Model file for the job. Use its own axes, mm. Face numbers are marked on the shaded views. Round coordinates to 2 decimals unless told otherwise and drop trailing zeros. Loops run counter-clockwise (first coordinate to the right, second up) from the corner with the lowest first, then second, coordinate; pieces in that order, holes last. Notation, with made-up numbers: (40.5, 69.5) - (89.5, 69.5) arc R29 cw to (89.5, 93.5) - close; hole circle Ø9 at (78.25, 79). An arc over 180 degrees is marked (long way). Answer as a JSON object with one key per item and string values.
Solid Edge part; units mm, degrees
sketch "Sketch1" plane through (0, 0, 0) normal (0, 0, 1) x (1, 0, 0)
  line L0 (15, -30) -> (-15, -30)
  line L1 (-15, -30) -> (-15, 30)
  line L2 (-15, 30) -> (15, 30)
  line L3 (15, 30) -> (15, -30)
extrude "Protrusion1" add sketch "Sketch1" against normal blind 5
sketch "Sketch2" plane through (0, -30, -2.5) normal (0, -1, 0) x (1, 0, 0)
  line L0 (15, -2.5) -> (15, -4.45)
  line L1 (15, -4.45) -> (-15, -4.45)
  line L2 (-15, -4.45) -> (-15, -2.5)
  line L3 (-15, -2.5) -> (15, -2.5)
extrude "ExtrudedProtrusion_2" add sketch "Sketch2" against normal blind 15
fillet "Round_1" radius 2 1 edges at (0, -15, -6.95)
sketch "Sketch3" plane through (0, -30, -3.475) normal (0, -1, 0) x (1, 0, 0)
  circle A0 centre (-5.74, -3.475) radius 0.5
  circle A1 centre (-2.87, -3.475) radius 0.5
  circle A2 centre (0, -3.475) radius 0.5
  circle A3 centre (2.87, -3.475) radius 0.5
  circle A4 centre (5.74, -3.475) radius 0.5
extrude "Cutout1" cut sketch "Sketch3" against normal up to next
sketch "Sketch4" plane through (0, 0, 0) normal (0, 0, 1) x (1, 0, 0)
  circle A0 centre (11.5, -25) radius 2.125
  circle A1 centre (-11.5, -25) radius 2.125
  circle A2 centre (-11.5, 25) radius 2.125
  circle A3 centre (11.5, 25) radius 2.125
extrude "Cutout2" cut sketch "Sketch4" against normal up to next
sketch "Sketch5" plane through (0, 7.5, -5) normal (0, 0, -1) x (-1, 0, 0)
  line L0 (3.2448, 10.1167) -> (3.2448, -2.3765)
  line L1 (3.2448, -2.3765) -> (8.2455, -2.3765)
  line L2 (8.2455, -2.3765) -> (8.2455, 10.1167)
  line L3 (8.2455, 10.1167) -> (3.2448, 10.1167)
extrude "Cutout3" cut sketch "Sketch5" against normal up to next
sketch "Sketch6" plane through (15, 0, -3.475) normal (1, 0, 0) x (0, 1, 0)
  line L0 (-15, -1.525) -> (-14.875, 3.475)
  line L1 (-14.875, 3.475) -> (30, 3.475)
  line L2 (30, 3.475) -> (30, -1.525)
  line L3 (30, -1.525) -> (-15, -1.525)
extrude "Cutout4" cut sketch "Sketch6" against normal up to next
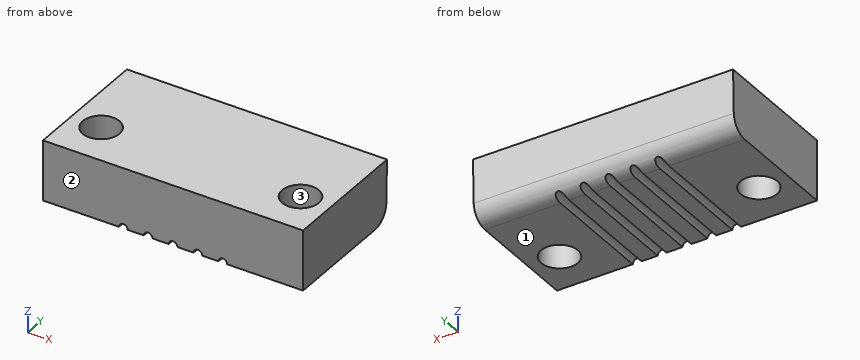
1) Two-plate mould, pull along Y, no slides. Class the marked faces 1, 2 and 3: pulls with the +Y half, pulls with the -Y half, needs draft (parallel to the pull), parting line crosses it, or undercut.
Values follow:
{"face 1": "needs draft", "face 2": "pulls with the -Y half", "face 3": "undercut"}
2) Slice it at A-A on y = -25. List the corners of the cut face in (x, z) (3 decimals).
Values follow:
{"outline": "(-15, -6.95) - (-13.625, -6.95) - (-13.625, 0) - (-15, 0) - close; (-9.375, -6.95) - (-6.24, -6.95) arc R0.5 cw to (-5.24, -6.95) - (-3.37, -6.95) arc R0.5 cw to (-2.37, -6.95) - (-0.5, -6.95) arc R0.5 cw to (0.5, -6.95) - (2.37, -6.95) arc R0.5 cw to (3.37, -6.95) - (5.24, -6.95) arc R0.5 cw to (6.24, -6.95) - (9.375, -6.95) - (9.375, 0) - (-9.375, 0) - close; (13.625, -6.95) - (15, -6.95) - (15, 0) - (13.625, 0) - close"}
3) Slice it at B-B on x = 11.5. List the corners of the cut face in (y, z) (3 decimals).
Values follow:
{"outline": "(-30, -6.95) - (-27.125, -6.95) - (-27.125, 0) - (-30, 0) - close; (-22.875, -6.95) - (-17, -6.95) arc R2 ccw to (-15, -4.95) - (-15, -5) - (-14.875, 0) - (-22.875, 0) - close"}
4) Slice it at C-C on z = -1.75. List the corners of the cut face in (x, y) (3 decimals), then the cut area to 3 significant figures.
Values follow:
{"outline": "(-15, -30) - (15, -30) - (15, -14.919) - (-15, -14.919) - close; hole circle Ø4.25 at (-11.5, -25); hole circle Ø4.25 at (11.5, -25)", "area": "424 mm²"}
5) Probe probe 1 along X at (y, z) = (-23.75, -3.5); probe 2 along Y at (x, z) = (-11.5, -5.25) (3 decimals); probe 3 along Y at (x, z) = (-11.5, -2.25) (3 decimals). List the from-to ranges inside material, lowest first.
Values follow:
{"probe 1": "-15 to -13.22, -9.78 to 9.78, 13.22 to 15", "probe 2": "-30 to -27.125, -22.875 to -15.023", "probe 3": "-30 to -27.125, -22.875 to -14.931"}
6) Slice it at D-D on x = 5.74. List the corners of the cut face in (y, z) (3 decimals), then the cut area to 3 significant figures.
Values follow:
{"outline": "(-30, -6.45) - (-15.677, -6.45) arc R2 ccw to (-15, -4.95) - (-15, -5) - (-14.875, 0) - (-30, 0) - close", "area": "96.8 mm²"}
